Check sheet for the modelled part. Datum: model origin and axes. Units: mm. Give positions to 0.01 mm unless a question says otherwise; leave off trailing zeros. Order: outer loops, then holes, each group sorted by start corner. A loop starts at its lowest first (then second) coordinate and runs counter-clockwise, first axis right, second up. Notation, with made-up numbers: (4.25, 82) - (11.25, 82) arc R17 ccw to (11.25, 91) - close; hole circle Ø6 at (25.5, -34). An arc over 180 degrees is marked (long way). Answer in a Markdown table with one row per item.
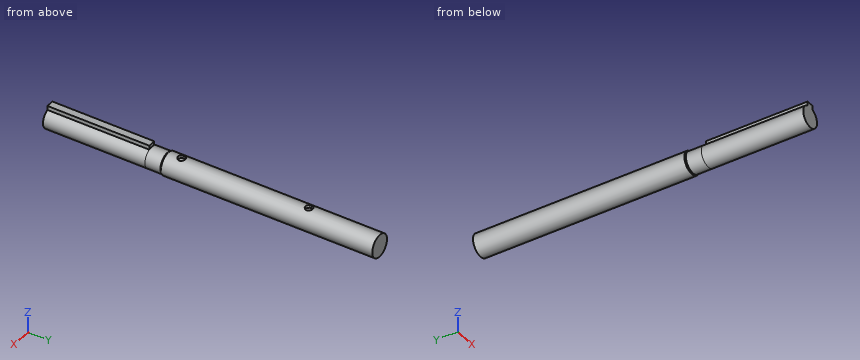
from build123d import *

# Parameters (mm, degrees)
F1_DEPTH    = 34
F2_R        = 7
F3_DEPTH    = 10
F4_R        = 7.5
F5_DEPTH    = 142
F7_R        = 2.5
F8_DEPTH    = 2
F9_S5_R     = 7
F9_T6_DEPTH = 12


# Not quite as in the source:
# - a fillet or chamfer that OpenCascade refuses, or shapes differently, is made with other operations: its cross-section is extruded or revolved along the edge and cut away or added
# - after a boolean that leaves OpenCascade's solid faulty, fix() repairs it


with BuildPart() as f1:
    # F0 (on Front) → F1 (new body, symmetric)
    with BuildSketch(Plane.XZ):
        with BuildLine():
            Line((-2.5, 9.3003484153), (-2.5, 6.5383484153))
            ThreePointArc((-2.5, 6.5383484153), (0, -7), (2.5, 6.5383484153))
            Line((2.5, 6.5383484153), (2.5, 9.3003484153))
            Line((2.5, 9.3003484153), (-2.5, 9.3003484153))
        make_face()
    extrude(amount=F1_DEPTH, both=True)

    # F2 (on face) → F3 (join)
    with BuildSketch(Plane(origin=(0, 34, 0), x_dir=(-1, 0, 0), z_dir=(0, 1, 0))):
        Circle(F2_R)
    extrude(amount=F3_DEPTH)

    # F4 (on face) → F5 (join)
    with BuildSketch(Plane(origin=(0, 44, 0), x_dir=(-1, 0, 0), z_dir=(0, 1, 0))):
        Circle(F4_R)
    extrude(amount=F5_DEPTH)

    add(f1.part.fix(), mode=Mode.REPLACE)

    # F7 (on offset) → F8 (cut)
    with BuildSketch(Plane.XY.offset(7.5)):
        with Locations((0, 54)):
            Circle(F7_R)
        with Locations((0, 139)):
            Circle(F7_R)
    extrude(amount=-F8_DEPTH, mode=Mode.SUBTRACT)

    # F9: chamfer of 1 on 1 edges, made by hand


with BuildPart() as f9_tool2:
    # F9_s3 → F9_t4 (revolve)
    with BuildSketch(Plane.XY):
        Polygon((-7.5, 45), (-6.5, 44), (-7.5, 44), align=None)
    revolve(axis=Axis((0, 44, 0), (0, 1, 0)))

    # F9_s5 → F9_t6 (cut, symmetric)
    with BuildSketch(Plane.XZ.offset(-44.5)):
        Circle(F9_S5_R)
    extrude(amount=F9_T6_DEPTH, both=True, mode=Mode.SUBTRACT)


with BuildPart() as f1_1:
    add(f1.part)

    # F9_t1: cut F9_tool2
    add(f9_tool2.part, mode=Mode.SUBTRACT)


solid = f1_1.part
(1) Cross-section at C-C, the plane y = 124. Record the cut outline in (x, z), then the cut area to 3 significant figures.
Geometry says:
| item | result |
|---|---|
| outline | circle Ø15 at (0, 0) |
| area | 177 mm² |
(2) Gauge pin test, flat ends, axial feed: P1, Ø2, axis at y = 6, z = -2, coming from the +X side; P2, Ø6, axis at y = 36.5, z = -3.5, coming from the -X side; P3, Ø0.8, axis at y = 16, z = 7.5, coming from the +X side. Record the tip position at first contact, or that the pin passes through.
Geometry says:
| item | result |
|---|---|
| P1 | x = 6.93 |
| P2 | x = -6.98 |
| P3 | x = 2.5 |
(3) Cross-section at B-B, the plane x = 0. Record the cut outline in (y, z).
Geometry says:
| item | result |
|---|---|
| outline | (-34, -7) - (44.5, -7) - (45, -7.5) - (186, -7.5) - (186, 7.5) - (141.5, 7.5) - (141.5, 5.5) - (136.5, 5.5) - (136.5, 7.5) - (56.5, 7.5) - (56.5, 5.5) - (51.5, 5.5) - (51.5, 7.5) - (45, 7.5) - (44.5, 7) - (34, 7) - (34, 9.3) - (-34, 9.3) - close |
(4) Cross-section at D-D, the plane y = -8. Record the cut outline in (x, z).
Geometry says:
| item | result |
|---|---|
| outline | (-2.5, 6.54) arc R7 ccw (long way) to (2.5, 6.54) - (2.5, 9.3) - (-2.5, 9.3) - close |
(5) Thickness scan on L1, parallel to Y at x = 0, z = 6.35; L2, parallel to Y at x = 2, z = 8; L3, parallel to X at y = 54, z = 6.7. Record the ranges inside material, lowest first.
Geometry says:
| item | result |
|---|---|
| L1 | -34 to 51.5, 56.5 to 136.5, 141.5 to 186 |
| L2 | -34 to 34 |
| L3 | -3.37 to -2.5, 2.5 to 3.37 |
(6) Cross-section at A-A, the plane z = 0. Record the cut outline in (x, y), then the cut area to 3 significant figures.
Geometry says:
| item | result |
|---|---|
| outline | (-7.5, 45) - (-7, 44.5) - (-7, -34) - (7, -34) - (7, 44.5) - (7.5, 45) - (7.5, 186) - (-7.5, 186) - close |
| area | 3,220 mm² |
